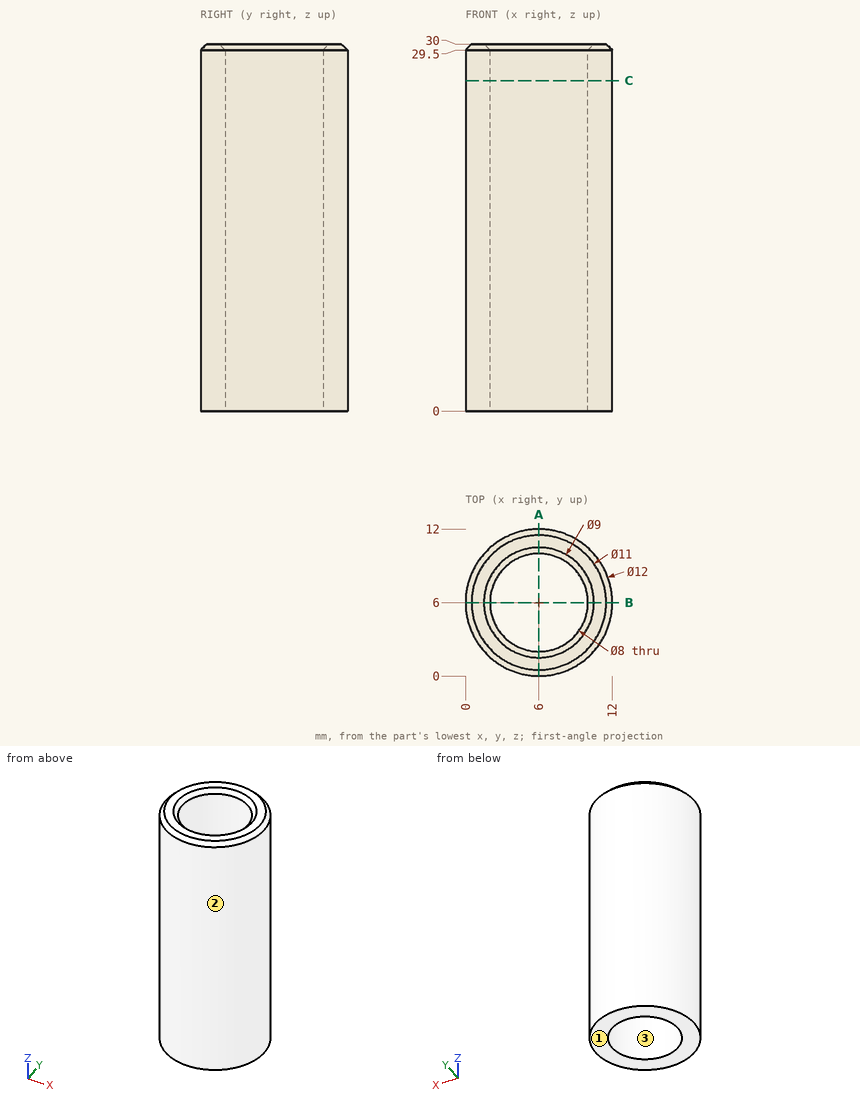
Study the drawing (mm; zero at the part's minimum x, y, z) and answer. Coordinates: 2 decimals unless noted, no trailing zeros. Order: outer loops, then holes, each group sorted by start corner. A loop starts at its lowest first (then second) coordinate and runs counter-clockwise, first axis right, second up. Notation, with made-up numbers: M 69,52.25 L 103,52.25 A21 cw 103,77.25 Z; hole C 45,34 d11. An arc over 180 degrees is marked long. Use CSV: the item, a comma, the result in double quotes.
Q1. Section A-A (x = 6) is taken. Determine the outline of the cut face in (y, z), then the cut area to 4 significant figures.
Here are the results:
outline,"M 0,0 L 2,0 L 2,29.5 L 1.5,30 L 0.5,30 L 0,29.5 Z; M 10,0 L 12,0 L 12,29.5 L 11.5,30 L 10.5,30 L 10,29.5 Z"
area,"119.5 mm2"
Q2. Straight lines are drawn through the part: L1, parallel to Y at x = 6, z = 10.25; L2, parallel to X at y = 8.5, z = 26.5; L3, parallel to Y at x = 5.25, z = 9.25. For each, find the intervals that lie inside material, in ascending order.
Here are the results:
L1,"0 to 2, 10 to 12"
L2,"0.55 to 2.88, 9.12 to 11.45"
L3,"0.05 to 2.07, 9.93 to 11.95"
Q3. Given pin 1 Ø6 at (x, y) = (9, 8.5) entering from +Z; pin 2 Ø6 at (y, z) = (2.5, 11.5) entering from +X; pin 3 Ø2 at (x, z) = (2, 20.5) entering from -Y; pin 4 Ø4 at (x, z) = (2, 8.5) entering from -Y, each flat-ended and moving along its own axis, determine where each tip first touches the part or whether it passes through.
Here are the results:
pin 1,"z = 30"
pin 2,"x = 11.98"
pin 3,"y = 0.8"
pin 4,"y = 0.34"
Q4. Section C-C (z = 27) is taken. Determine the outline of the cut face in (x, y), then the cut area to 3 significant figures.
Here are the results:
outline,"C 6,6 d12; hole C 6,6 d8"
area,"62.8 mm2"
Q5. Determine the mould class of the marked faces 1, 2 and 3 for opening direction Y: pulls with the +Y half, pulls with the -Y half, needs draft (parallel to the pull), parting line crosses it, or undercut.
Here are the results:
face 1,"needs draft"
face 2,"parting line crosses it"
face 3,"undercut"
